Verification items for this drawing (mm, ordinates from the low corner). Give positions to 0.01 mm unless a question says otherwise; leave off trailing zeros. Loops run counter-clockwise (first coordinate to the right, second up) from the corner with the lowest first, then second, coordinate; pieces in that order, holes last. Notation, with made-up numbers: M 55,-11 L 110,-11 A21 cw 110,15 Z; hole C 27.5,4.5 d7. An arc over 180 degrees is marked long. Use a Markdown table: item, result.
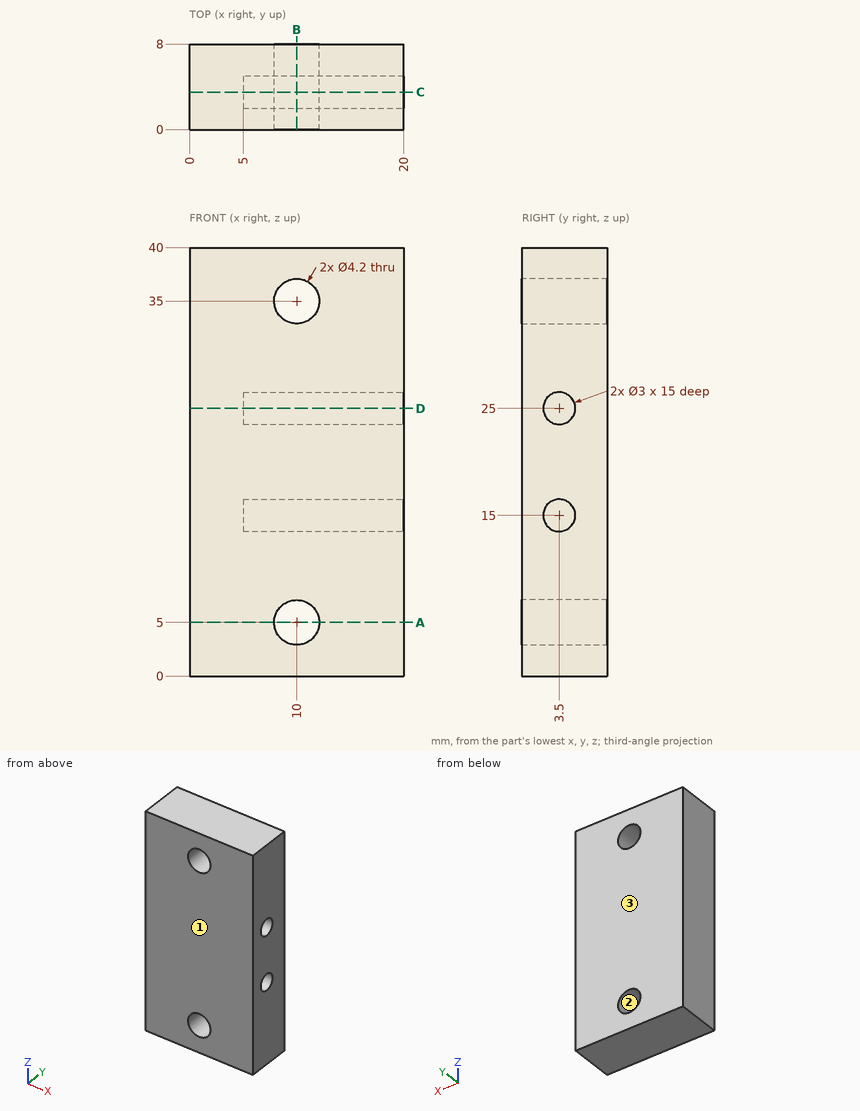
(1) Cross-section at D-D on z = 25. Record the cut outline in (x, y).
Results below:
| item | result |
|---|---|
| outline | M 0,0 L 20,0 L 20,2 L 5,2 L 5,5 L 20,5 L 20,8 L 0,8 Z |
(2) Cross-section at C-C on y = 3.5. Record the cut outline in (x, z).
Results below:
| item | result |
|---|---|
| outline | M 0,0 L 20,0 L 20,13.5 L 5,13.5 L 5,16.5 L 20,16.5 L 20,23.5 L 5,23.5 L 5,26.5 L 20,26.5 L 20,40 L 0,40 Z; hole C 10,5 d4.2; hole C 10,35 d4.2 |
(3) Draft check along Y on the marked faces 1, 2 and 3. Enter one of: +Y half, -Y half, draft (parallel to the pull), parting line (faces both ways), or undercut.
Results below:
| item | result |
|---|---|
| face 1 | -Y half |
| face 2 | draft |
| face 3 | +Y half |
(4) Cross-section at A-A on z = 5. Record the cut outline in (x, y).
Results below:
| item | result |
|---|---|
| outline | M 0,0 L 7.9,0 L 7.9,8 L 0,8 Z; M 12.1,0 L 20,0 L 20,8 L 12.1,8 Z |
(5) Gauge pin test, flat ends, axial feed: P1, Ø6.5, axis at x = 10, z = 5, coming from the -Y side; P2, Ø2.5, axis at y = 3.5, z = 15, coming from the +X side. Record the tip position at first contact, or that the pin passes through.
Results below:
| item | result |
|---|---|
| P1 | y = 0 |
| P2 | x = 5 |
(6) Cross-section at B-B on x = 10. Record the cut outline in (y, z).
Results below:
| item | result |
|---|---|
| outline | M 0,0 L 8,0 L 8,2.9 L 0,2.9 Z; M 0,7.1 L 8,7.1 L 8,32.9 L 0,32.9 Z; M 0,37.1 L 8,37.1 L 8,40 L 0,40 Z; hole C 3.5,15 d3; hole C 3.5,25 d3 |
(7) Material ranges on line 1 (X direction, y = 2, z = 35); line 2 (Z direction, x = 10.5, y = 1); line 3 (Z direction, x = 11, y = 3.5), recorded low to high.
Results below:
| item | result |
|---|---|
| line 1 | 0 to 7.9, 12.1 to 20 |
| line 2 | 0 to 2.96, 7.04 to 32.96, 37.04 to 40 |
| line 3 | 0 to 3.15, 6.85 to 13.5, 16.5 to 23.5, 26.5 to 33.15, 36.85 to 40 |
